```python
from build123d import *

# Parameters (mm, degrees)
CROQUIS_LENGUETA_BUJE_R        = 6
LENGUETA_BUJE_DEPTH            = 3
CROQUIS_LENGUETA_W             = 18
CROQUIS_LENGUETA_H             = 12
LENGUETA_DEPTH                 = 3
CROQUIS_CEJA_W                 = 60
CROQUIS_CEJA_H                 = 45
CEJA_MONITOR_DEPTH             = 12
AGUJERO_TRIPODE_1_4_DEPTH      = 69.242215673
AGUJERO_TRIPODE_1_4_DEPTH_BACK = 69.242215673
CROQUIS_ROSCA_R                = 3.25
EJE_M4_DEPTH                   = 69.242215673
EJE_M4_DEPTH_BACK              = 69.242215673
CROQUIS_EJE_R                  = 2.2


with BuildPart() as part:
    # Croquis_lengueta_buje → Lengueta_buje (new, symmetric)
    with BuildSketch(Plane(origin=(0, 0, 0), x_dir=(0, 0, -1), z_dir=(1, 0, 0))):
        Circle(CROQUIS_LENGUETA_BUJE_R)
    extrude(amount=LENGUETA_BUJE_DEPTH, both=True)

    # Croquis_lengueta → Lengueta (add, symmetric)
    with BuildSketch(Plane(origin=(0, 0, 0), x_dir=(0, 0, -1), z_dir=(1, 0, 0))):
        with Locations((-9, 0)):
            Rectangle(CROQUIS_LENGUETA_W, CROQUIS_LENGUETA_H)
    extrude(amount=LENGUETA_DEPTH, both=True)

    # Croquis_ceja → Ceja_monitor (add)
    with BuildSketch(Plane(origin=(0, -6, 0), x_dir=(1, 0, 0), z_dir=(0, 1, 0))):
        with Locations((0, -38.5)):
            Rectangle(CROQUIS_CEJA_W, CROQUIS_CEJA_H)
    extrude(amount=CEJA_MONITOR_DEPTH)

    # Croquis_rosca → Agujero_tripode_1_4 (cut, two sides: drawn at the far end of the back side and taken through both)
    with BuildSketch(Plane(origin=(0, 0, 0), x_dir=(1, 0, 0), z_dir=(0, 1, 0)).offset(-AGUJERO_TRIPODE_1_4_DEPTH_BACK)):
        with Locations(Location((0, -40, 0), (0, 0, 270))):
            Circle(CROQUIS_ROSCA_R)
    extrude(amount=AGUJERO_TRIPODE_1_4_DEPTH + AGUJERO_TRIPODE_1_4_DEPTH_BACK, mode=Mode.SUBTRACT)

    # Croquis_eje → Eje_M4 (cut, two sides: drawn at the far end of the back side and taken through both)
    with BuildSketch(Plane(origin=(0, 0, 0), x_dir=(0, 0, -1), z_dir=(1, 0, 0)).offset(-EJE_M4_DEPTH_BACK)):
        Circle(CROQUIS_EJE_R)
    extrude(amount=EJE_M4_DEPTH + EJE_M4_DEPTH_BACK, mode=Mode.SUBTRACT)


solid = part.part
```
The listing builds one solid part. Answer for the finished solid, in the listing's coordinates (mm). A direction names the side the tool comes from. Give positions to 0.01 mm unless a question says otherwise; leave off trailing zeros. Order: outer loops, then holes, each group sorted by start corner. A loop starts at its lowest first (then second) coordinate and runs counter-clockwise, first axis right, second up. Notation, with made-up numbers: (-28.75, -29) -> (12.25, -29) arc R17 ccw to (12.25, -22) -> close; hole circle Ø9 at (10, -32). An arc over 180 degrees is marked (long way). Answer as a JSON object with one key per item and string values. Group by question number.
Item 1: The part is cut by section C-C on y = -4.5. Write down the section's boundary in (x, z).
Item 2: Determine the mould class of faces 4 (the cylindrical face through (-1.245, -0.084, 43.002)), 5 (the flat face through (3, 0, 5)), 6 (the cylindrical face through (0, 0, -6)), 7 (the cylindrical face through (-0.04, 0.66, -2.1)) for opening direction Z: pulls with the +Z half, pulls with the -Z half, needs draft (parallel to the pull), parting line crosses it, or undercut.
Item 3: The part is cut by section A-A on y = 0. Write down the section's boundary in (x, z).
Item 4: The part is cut by section B-B on z = 41. Write down the section's boundary in (x, y), and give its area (3 significant figures).
Item 5: The part is cut by section D-D on x = -23. Write down the section's boundary in (y, z).
Item 6: A tool of negligible diameter and unlimited length cuts with its end or side. For faces 1 (the flat face through (16, 0, 16)), 2 (the flat face through (-17, 0, 16)), 3 (the flat face through (-30, 0, 39)), from which of +Z, -Z, +X, -X, +Y, -Y can it reach the whole face along a straight path? Write none if from no direction.
Item 7: Flat-ended cylindrical pins translate along their axes: pin 1 (6 mm diameter, centred on x = 10.5, y = 0, fed in from -Z); pin 2 (3.5 mm diameter, centred on y = -1, z = 3, fed in from +X). Find the tip coordinate at first contact, or state that the pin passes through.
Item 8: Consider L1, parallel to X at y = 2.75, z = 40; L2, parallel to Z at x = 0, y = -0.25; L3, parallel to Y at x = 0.15, z = 0. Determine where each line is inside the solid, lowest interval first. Write a range as from..to.
Result set:
{
 "1": {"outline": "(-30, 16) -> (-3, 16) -> (-3, -3.97) -> (3, -3.97) -> (3, 16) -> (30, 16) -> (30, 61) -> (-30, 61) -> close; hole circle Ø6.5 at (0, 40)"},
 "2": {"face 4": "undercut", "face 5": "needs draft", "face 6": "pulls with the -Z half", "face 7": "undercut"},
 "3": {"outline": "(-30, 16) -> (-3, 16) -> (-3, 2.2) -> (3, 2.2) -> (3, 16) -> (30, 16) -> (30, 61) -> (-30, 61) -> close; (-3, -6) -> (3, -6) -> (3, -2.2) -> (-3, -2.2) -> close; hole circle Ø6.5 at (0, 40)"},
 "4": {"outline": "(-30, -6) -> (-3.09, -6) -> (-3.09, 6) -> (-30, 6) -> close; (3.09, -6) -> (30, -6) -> (30, 6) -> (3.09, 6) -> close", "area": "646 mm²"},
 "5": {"outline": "(-6, 16) -> (6, 16) -> (6, 61) -> (-6, 61) -> close"},
 "6": {"face 1": "-Z, +X, +Y, -Y", "face 2": "-Z, -X, +Y, -Y", "face 3": "+Z, -Z, -X, +Y, -Y"},
 "7": {"pin 1": "z = 16", "pin 2": "x = 3"},
 "8": {"L1": "-30..-3.25, 3.25..30", "L2": "-5.99..-2.19, 2.19..36.75, 43.25..61", "L3": "-6..-2.2, 2.2..6"}
}
